Autodesk Inventor part; units mm, degrees
ref_plane "YZ Plane" through (0, 0, 0) normal (1, 0, 0) x (0, 1, 0)
ref_plane "XZ Plane" through (0, 0, 0) normal (0, 1, 0) x (-1, 0, 0)
ref_plane "XY Plane" through (0, 0, 0) normal (0, 0, 1) x (1, 0, 0)
sketch "Skizze1" plane through (0, 0, 0) normal (1, 0, 0) x (0, 1, 0)
  circle A0 centre (0, 0) radius 40
  circle A1 centre (0, 0) radius 108
  dimension "d0" = 216
  dimension "d1" = 80
extrude "Extrusion1" add sketch "Skizze1" along normal blind 15
sketch "Skizze2" plane through (15, 0, 0) normal (1, 0, 0) x (0, 0, -1)
  circle A0 centre (0, 0) radius 40
  circle A1 centre (0, 0) radius 50
  dimension "d4" = 100
extrude "Extrusion2" add sketch "Skizze2" along normal blind 235
fillet "Rundung1" radius 10 1 edges at (15, 0, 50)
sketch "Skizze3" plane through (15, 0, 0) normal (1, 0, 0) x (0, 0, -1)
  circle A0 centre (0, -85) radius 10 construction
  line L0 (0, -95) -> (-8.7647, -89.8146)
  line L1 (-8.7647, -80.1854) -> (0, -75)
  line L2 (0, -75) -> (8.7647, -80.1854)
  line L3 (8.7647, -80.1854) -> (8.7647, -89.8146)
  line L4 (0, -95) -> (8.7647, -89.8146)
  line L5 (-8.7647, -80.1854) -> (-8.7647, -89.8146)
  point P0 (0, 0)
  dimension "d8" = 20
  dimension "d9" = 85
extrude "Extrusion3" add sketch "Skizze3" along normal blind 10
sketch "Skizze4" plane through (25, 0, 0) normal (1, 0, 0) x (0, 0, -1)
  circle A0 centre (0, -85) radius 5
  point P0 (0, 0)
  dimension "d12" = 10
extrude "Extrusion4" add sketch "Skizze4" along normal blind 10
pattern_circular "Runde Anordnung1" count 6 over 360 about axis through (-10, 0, 0) along (1, 0, 0) of "Extrusion3", "Extrusion4"
mirror "Spiegeln1" about plane through (250, 0, 0) normal (1, 0, 0) of "Extrusion3", "Extrusion4", "Runde Anordnung1", "Extrusion2", "Extrusion1", "Rundung1"
properties part number "DN80-05m"
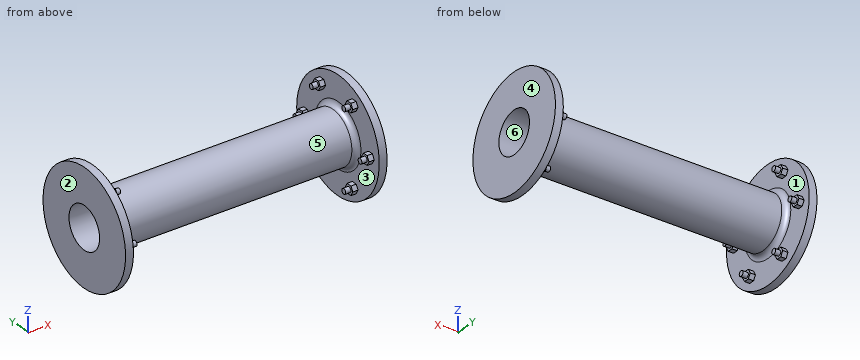
Geometry: final body of the model. Coordinates: model frame, mm. Face numbers are marked on the shaded views. A direction names the side the tool comes from. Coordinates: 2 decimals unless noted, no trailing zeros. Order: outer loops, then holes, each group sorted by start corner. A loop starts at its lowest first (then second) coordinate and runs counter-clockwise, first axis right, second up. Notation, with made-up numbers: (58.5, 89) - (115.5, 89) arc R12 ccw to (115.5, 93) - close; hole circle Ø6 at (17, 50). An arc over 180 degrees is marked (long way). Return JSON: item names as keys, results as strings. Group by question number.
1. Pull-direction query (X, two-part tool) for the marked faces 1, 2, 3 and 4; classes: pulls with the +X half, pulls with the -X half, needs draft (parallel to the pull), parting line crosses it, or undercut.
2. Pin query (flat end, axial travel): pin 1 (12 mm diameter, centred on x = 415.5, y = -49.5, fed in from +Z); pin 2 (8 mm diameter, centred on y = 85, z = 0.5, fed in from -X); pin 3 (5 mm diameter, centred on x = 422, z = 48.5, fed in from -Y); pin 4 (3 mm diameter, centred on x = 18, y = 86, fed in from -Z). Return the tip coordinate at first contact, or that it passes through.
3. Cut plane A-A (y = 0). Output: boundary loops of the cut face in (x, z).
4. Set-up query: the marked faces 5 and 6. Return all of +Z, -Z, +X, -X, +Y, -Y with unobstructed straight access to the full face (end or side cutting, diameter ignored); none if empty.
5. Material intervals for line 1 along X through (y, z) = (71.5, 15); line 2 along Z through (x, y) = (444, -22.5); line 3 along Y through (x, z) = (295, 22), sorted ascending. Write a range as [from, to].
6. Cut plane C-C (x = 384). Output: boundary loops of the cut face in (y, z).
7. Cut plane D-D (y = 85). Output: boundary loops of the cut face in (x, z).
8. Cut plane B-B (z = 94). Output: boundary loops of the cut face in (x, y), plus the area to 3 significant figures.
Resolved:
{
 "1": {"face 1": "undercut", "face 2": "pulls with the -X half", "face 3": "undercut", "face 4": "pulls with the +X half"},
 "2": {"pin 1": "stops at z = 24.65", "pin 2": "stops at x = 0", "pin 3": "stops at y = -19.6", "pin 4": "stops at z = -8.76"},
 "3": {"outline": "(0, -108) - (15, -108) - (15, -60) arc R10 cw to (25, -50) - (475, -50) arc R10 cw to (485, -60) - (485, -108) - (500, -108) - (500, -40) - (0, -40) - close; (0, 40) - (500, 40) - (500, 108) - (485, 108) - (485, 60) arc R10 cw to (475, 50) - (25, 50) arc R10 cw to (15, 60) - (15, 108) - (0, 108) - close"},
 "4": {"face 5": "none", "face 6": "+X, -X"},
 "5": {"line 1": "x = [0, 15], [485, 500]", "line 2": "z = [-44.65, -33.07], [33.07, 44.65]", "line 3": "y = [-44.9, -33.41], [33.41, 44.9]"},
 "6": {"outline": "circle Ø100 at (0, 0); hole circle Ø80 at (0, 0)"},
 "7": {"outline": "(0, -66.63) - (15, -66.63) - (15, -8.76) - (25, -8.76) - (25, -5) - (35, -5) - (35, 5) - (25, 5) - (25, 8.76) - (15, 8.76) - (15, 66.63) - (0, 66.63) - close; (465, -5) - (475, -5) - (475, -8.76) - (485, -8.76) - (485, -66.63) - (500, -66.63) - (500, 66.63) - (485, 66.63) - (485, 8.76) - (475, 8.76) - (475, 5) - (465, 5) - close"},
 "8": {"outline": "(0, -53.18) - (15, -53.18) - (15, 53.18) - (0, 53.18) - close; (485, -53.18) - (500, -53.18) - (500, 53.18) - (485, 53.18) - close", "area": "3,190 mm²"}
}
